Check sheet for the drawn part. Datum: minimum x, y, z corner. Units: mm. A direction names the side the tool comes from. Round coordinates to 2 decimals unless told otherwise and drop trailing zeros. Write each loop counter-clockwise with the first axis right and the second up, starting at its lowest first coordinate (ties: lowest second). Pieces come first, ordered by that corner, then holes. Notation, with made-up numbers: (48, 14) -> (55, 14) arc R37 cw to (55, 53) -> close; hole circle Ø9 at (76.25, 85). An arc over 180 degrees is marked (long way). Use a Markdown table: item, result.
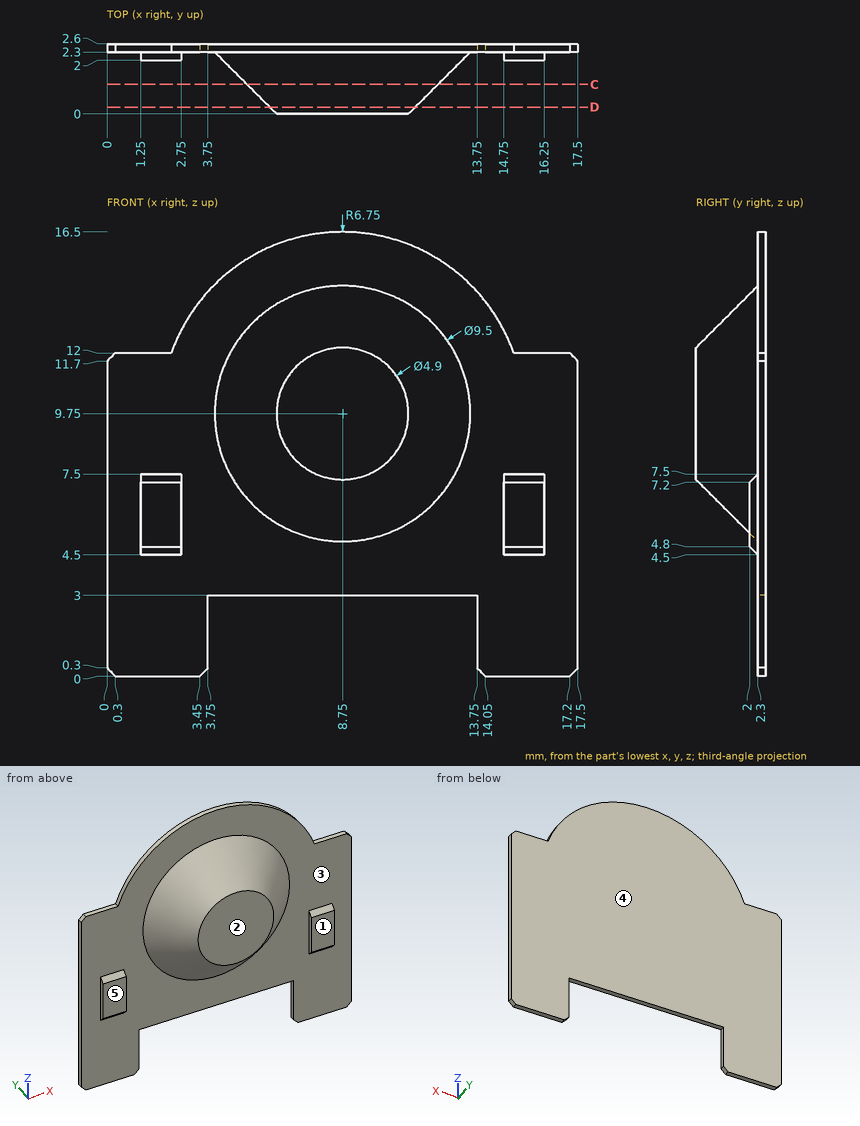
(1) Thickness scan on line 1 (Y direction, x = 12, z = 14.25); line 2 (Z direction, x = 8, y = 1.3); line 3 (X direction, y = 1.65, z = 12.75). Record the ranges inside material, lowest first.
A:
| item | result |
|---|---|
| line 1 | y = 2.3 to 2.6 |
| line 2 | z = 6.08 to 13.42 |
| line 3 | x = 5.96 to 11.54 |
(2) Section check C-C on y = 1.1. Record the cut outline in (x, z), plus the area to 3 significant figures.
A:
| item | result |
|---|---|
| outline | circle Ø7.1 at (8.75, 9.75) |
| area | 39.6 mm2 |
(3) Gauge pin test, flat ends, axial feed: pin 1 Ø1.6 at (x, z) = (15.5, 5.5) entering from -Y; pin 2 Ø5 at (x, z) = (15, 10.5) entering from -Y; pin 3 Ø1 at (x, z) = (15.5, 11) entering from -Y. Record the tip position at first contact, or that the pin passes through.
A:
| item | result |
|---|---|
| pin 1 | stops at y = 2 |
| pin 2 | stops at y = 1.34 |
| pin 3 | stops at y = 2.3 |
(4) Section check D-D on y = 0.25. Record the cut outline in (x, z), plus the area to 3 significant figures.
A:
| item | result |
|---|---|
| outline | circle Ø5.4 at (8.75, 9.75) |
| area | 22.9 mm2 |
(5) Access from +Z, -Z, +X, -X, +Y, -Y to the whole of each face (thin tool, end or side, straight path). Record for the marked faces 1, 2, 3, 4 and 5.
A:
| item | result |
|---|---|
| face 1 | +Z, -Z, +X, -Y |
| face 2 | +Z, -Z, +X, -X, -Y |
| face 3 | -Y |
| face 4 | +Z, -Z, +X, -X, +Y |
| face 5 | +Z, -Z, -X, -Y |
